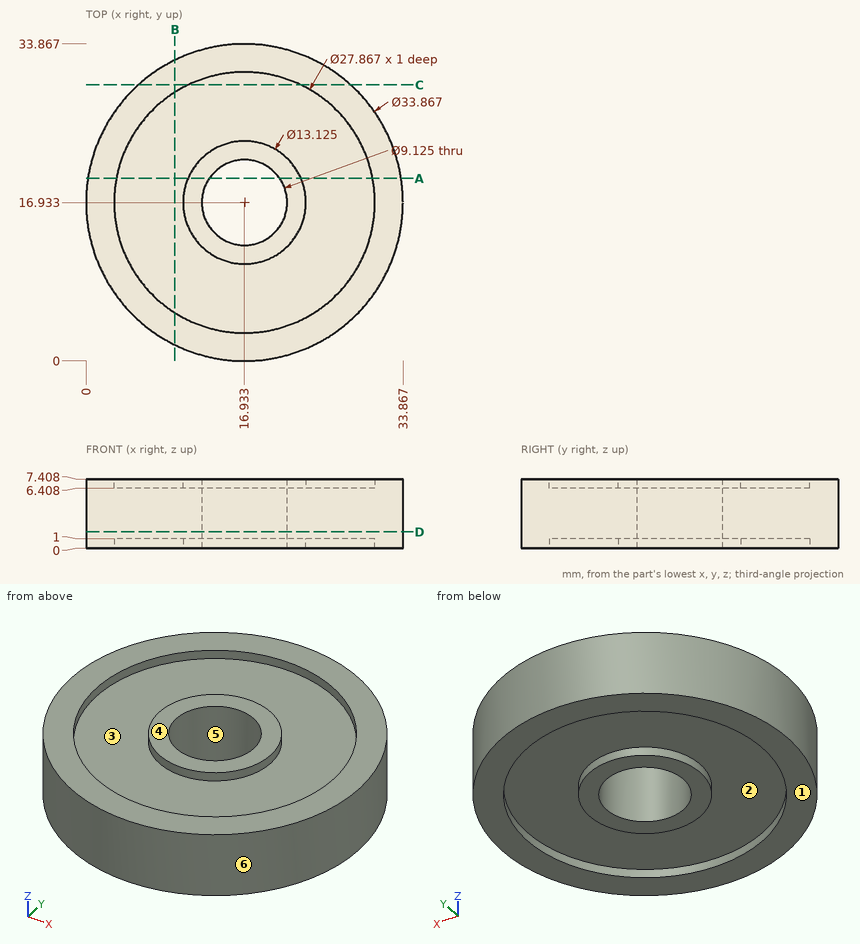
Study the drawing (mm; zero at the part's minimum x, y, z) and answer. A direction names the side the tool comes from. Round coordinates to 2 decimals unless told otherwise and drop trailing zeros. Write each loop counter-clockwise with the first axis right and the second up, starting at its lowest first coordinate (ties: lowest second). Pieces come first, ordered by that corner, then holes. Notation, with made-up numbers: (83.5, 66.5) - (108.5, 66.5) arc R10 cw to (108.5, 79.5) - close; hole circle Ø6 at (6, 25). An arc over 180 degrees is marked (long way). Use a Markdown table: item, result. Add a question column.
1. The part is cut by section A-A (y = 19.5). Write down the section's boundary in (x, z) (1 decimal).
2. Consider line 1 (Y direction, x = 18.5, z = 6.5) (1 decimal); line 2 (Z direction, x = 22.5, y = 6.5); line 3 (Y direction, x = 22.5, z = 0.75) (1 decimal). Determine where each line is inside the solid, lowest interval first.
3. For a pull along X with two mould halves and no side action, classify the marked faces 4, 5 and 6 as +X half, -X half, draft (parallel to the pull), parting line (faces both ways), or undercut.
4. The part is cut by section C-C (y = 29.5). Write down the section's boundary in (x, z) (1 decimal).
5. The part is cut by section B-B (x = 9.5). Write down the section's boundary in (y, z).
6. The part is cut by section D-D (z = 1.75). Write down the section's boundary in (x, y) (1 decimal).
7. A tool of negligible diameter and unlimited length cuts with its end or side. For the marked faces 1, 2 and 3, from which of +Z, -Z, +X, -X, +Y, -Y can it reach the whole face along a straight path? Write none if from no direction.
8. Flat-ended cylindrical pins translate along their axes: P1, Ø1, axis at x = 16, z = 6, coming from the +Y side; P2, Ø1, axis at x = 12.5, y = 24, coming from the -Z side; P3, Ø2, axis at x = 24.5, z = 6.5, coming from the +Y side. Find the tip coordinate at first contact, or state that the pin passes through.
Reported:
| question | item | result |
|---|---|---|
| 1 | outline | (0.2, 0) - (3.2, 0) - (3.2, 1) - (10.9, 1) - (10.9, 0) - (13.2, 0) - (13.2, 7.4) - (10.9, 7.4) - (10.9, 6.4) - (3.2, 6.4) - (3.2, 7.4) - (0.2, 7.4) - close; (20.7, 0) - (23, 0) - (23, 1) - (30.6, 1) - (30.6, 0) - (33.7, 0) - (33.7, 7.4) - (30.6, 7.4) - (30.6, 6.4) - (23, 6.4) - (23, 7.4) - (20.7, 7.4) - close |
| 2 | line 1 | 0.1 to 3.1, 10.6 to 12.6, 21.2 to 23.3, 30.8 to 33.8 |
| 2 | line 2 | 1 to 6.41 |
| 2 | line 3 | 0.9 to 4.2, 13.5 to 20.4, 29.7 to 32.9 |
| 3 | face 4 | draft |
| 3 | face 5 | undercut |
| 3 | face 6 | parting line |
| 4 | outline | (5.6, 0) - (10.9, 0) - (10.9, 1) - (23, 1) - (23, 0) - (28.3, 0) - (28.3, 7.4) - (23, 7.4) - (23, 6.4) - (10.9, 6.4) - (10.9, 7.4) - (5.6, 7.4) - close |
| 5 | outline | (1.72, 0) - (5.15, 0) - (5.15, 1) - (28.72, 1) - (28.72, 0) - (32.15, 0) - (32.15, 7.41) - (28.72, 7.41) - (28.72, 6.41) - (5.15, 6.41) - (5.15, 7.41) - (1.72, 7.41) - close |
| 6 | outline | circle Ø33.9 at (16.9, 16.9); hole circle Ø9.1 at (16.9, 16.9) |
| 7 | face 1 | -Z, +X, -X, +Y, -Y |
| 7 | face 2 | -Z |
| 7 | face 3 | +Z |
| 8 | P1 | y = 33.86 |
| 8 | P2 | z = 1 |
| 8 | P3 | y = 32.54 |
